from build123d import *

# Parameters (mm, degrees)
F0_R     = 32
F1_DEPTH = 10
F3_DEPTH = 2.1
F5_DEPTH = 25


with BuildPart() as f1:
    # F0 (on Top) → F1 (new body)
    with BuildSketch(Plane.XY):
        Circle(F0_R)
        with BuildLine():
            ThreePointArc((-1.5, -28.961181), (-29, 0), (-1.5, 28.961181))
            Line((-1.5, 28.961181), (-1.5, -28.961181))
        make_face(mode=Mode.SUBTRACT)
        with BuildLine():
            ThreePointArc((1.5, 28.961181), (29, 0), (1.5, -28.961181))
            Line((1.5, -28.961181), (1.5, 28.961181))
        make_face(mode=Mode.SUBTRACT)
    extrude(amount=F1_DEPTH)

    # F2 (on face) → F3 (join)
    with BuildSketch(Plane.XY.offset(10)):
        with BuildLine():
            Line((20.141127, 6), (36.510273, 6))
            ThreePointArc((36.510273, 6), (-37, 0), (36.510273, -6))
            Line((36.510273, -6), (20.141127, -6))
            ThreePointArc((20.141127, -6), (14.141127, 0), (20.141127, 6))
        make_face()
    extrude(amount=F3_DEPTH)

    # F4 (on face) → F5 (cut)
    with BuildSketch(Plane.XY.offset(10)):
        with BuildLine():
            Line((36.510273, 6), (20.141127, 6))
            ThreePointArc((20.141127, 6), (14.141127, 0), (20.141127, -6))
            Line((20.141127, -6), (36.510273, -6))
            Line((36.510273, -6), (36.510273, 6))
        make_face()
    extrude(amount=-F5_DEPTH, mode=Mode.SUBTRACT)


solid = f1.part
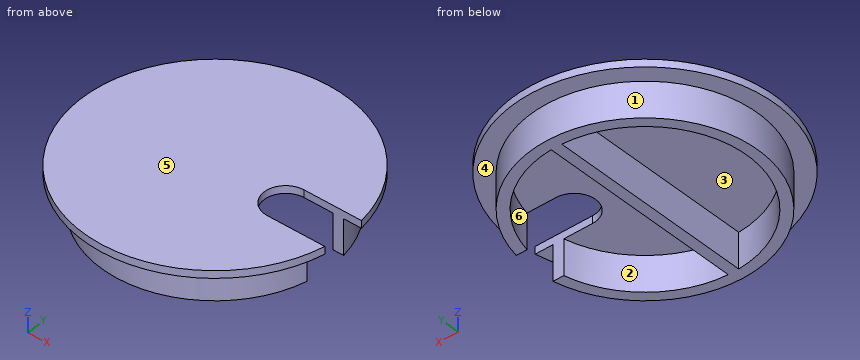
Design review of the part built by this model. Coordinates are the model's own, in mm. Face numbers are marked on the shaded views. A direction names the side the tool comes from. Give positions to 0.01 mm unless a question says otherwise; leave off trailing zeros. Loops run counter-clockwise (first coordinate to the right, second up) from the corner with the lowest first, then second, coordinate; pieces in that order, holes last. Notation, with made-up numbers: (32.5, -2) - (71.5, -2) arc R25 ccw to (71.5, 11) - close; hole circle Ø7 at (-9, 43). An arc over 180 degrees is marked (long way). Write item = value, one per line.
1) Take a section at D-D on x = -20. State the section outline as (y, z) points.
Result sheet:
outline = (-31.13, 10) - (-24.98, 10) - (-24.98, 0) - (-21, 0) - (-21, 10) - (21, 10) - (21, 0) - (24.98, 0) - (24.98, 10) - (31.13, 10) - (31.13, 12.1) - (-31.13, 12.1) - close
2) Take a section at B-B on x = 0. State the section outline as (y, z) points.
Result sheet:
outline = (-37, 10) - (-32, 10) - (-32, 0) - (32, 0) - (32, 10) - (37, 10) - (37, 12.1) - (-37, 12.1) - close
3) Clearance check with flat-ended pins moving along their axes: pin 1 Ø8 at (x, y) = (12.5, 10) entering from -Z; pin 2 Ø6 at (y, z) = (25, 6) entering from +X; pin 3 Ø2 at (y, z) = (-9.5, 1.5) entering from -X. State where each tip first meets the part, or that it passes through.
Result sheet:
pin_1 = 10
pin_2 = 23.24
pin_3 = -30.85
4) Draft analysis for pull direction Y (two halves, no side actions). For the marked faces 1, 2, 3 and 4, state which applies: +Y half, -Y half, draft (parallel to the pull), parting line (faces both ways), or undercut.
Result sheet:
face_1 = parting line
face_2 = undercut
face_3 = undercut
face_4 = draft
5) To check wall thickness, follow line 1 (X direction, y = 17.5, z = 0.5); line 2 (X direction, y = -21.5, z = 6); line 3 (Z direction, x = 2, y = 3). State the ranges of each line that lie inside material, in increasing order.
Result sheet:
line_1 = -26.79 to -23.12, -1.5 to 1.5, 23.12 to 26.79
line_2 = -23.7 to -19.46, -1.5 to 1.5, 19.46 to 23.7
line_3 = 10 to 12.1
6) Take a section at A-A on z = 8. State the section outline as (x, y) points, and give its area (3 significant figures).
Result sheet:
outline = (1.5, -28.96) - (1.5, 28.96) arc R29 cw to (28.37, 6) - (31.43, 6) arc R32 ccw (long way) to (31.43, -6) - (28.37, -6) arc R29 cw to start; hole (-1.5, -28.96) - (-1.5, 28.96) arc R29 ccw to start
area = 713 mm2
7) Tool access review of the marked faces 5 and 6: name each direction out of +Z, -Z, +X, -X, +Y, -Y from which nothing blocks a thin tool from reaching the whole face with its end or side.
Result sheet:
face_5 = +Z, +X, -X, +Y, -Y
face_6 = -Z
8) Take a section at C-C on y = 0. State the section outline as (x, z) points, and give its area (3 significant figures).
Result sheet:
outline = (-37, 10) - (-32, 10) - (-32, 0) - (-29, 0) - (-29, 10) - (-1.5, 10) - (-1.5, 0) - (1.5, 0) - (1.5, 10) - (14.14, 10) - (14.14, 12.1) - (-37, 12.1) - close
area = 167 mm2
